from build123d import *

# Parameters (mm, degrees)
BOSS_EXTRUDE1_DEPTH = 2.3
CUT_EXTRUDE1_REACH  = 4.3
SKETCH2_R           = 2.65
SKETCH2_R_2         = 5.125


with BuildPart() as part:
    # Sketch1 → Boss-Extrude1 (new body)
    with BuildSketch(Plane.XY):
        with BuildLine():
            Line((40.15, 0), (-40.15, 0))
            ThreePointArc((-40.15, 0), (-47.221067812, 2.928932188), (-50.15, 10))
            Line((-50.15, 10), (-50.15, 10.4))
            ThreePointArc((-50.15, 10.4), (-47.221067812, 17.471067812), (-40.15, 20.4))
            Line((-40.15, 20.4), (-24.25, 20.4))
            ThreePointArc((-24.25, 20.4), (-20.714466094, 21.864466094), (-19.25, 25.4))
            Line((-19.25, 25.4), (-19.25, 27.1))
            ThreePointArc((-19.25, 27.1), (-20.714466094, 30.635533906), (-24.25, 32.1))
            Line((-24.25, 32.1), (-31.13, 32.1))
            ThreePointArc((-31.13, 32.1), (-34.665533906, 33.564466094), (-36.13, 37.1))
            Line((-36.13, 37.1), (-36.13, 37.6))
            ThreePointArc((-36.13, 37.6), (-34.665533906, 41.135533906), (-31.13, 42.6))
            Line((-31.13, 42.6), (31.13, 42.6))
            ThreePointArc((31.13, 42.6), (34.665533906, 41.135533906), (36.13, 37.6))
            Line((36.13, 37.6), (36.13, 37.1))
            ThreePointArc((36.13, 37.1), (34.665533906, 33.564466094), (31.13, 32.1))
            Line((31.13, 32.1), (24.25, 32.1))
            ThreePointArc((24.25, 32.1), (20.714466094, 30.635533906), (19.25, 27.1))
            Line((19.25, 27.1), (19.25, 25.4))
            ThreePointArc((19.25, 25.4), (20.714466094, 21.864466094), (24.25, 20.4))
            Line((24.25, 20.4), (40.15, 20.4))
            ThreePointArc((40.15, 20.4), (47.221067812, 17.471067812), (50.15, 10.4))
            Line((50.15, 10.4), (50.15, 10))
            ThreePointArc((50.15, 10), (47.221067812, 2.928932188), (40.15, 0))
        make_face()
    extrude(amount=BOSS_EXTRUDE1_DEPTH)

    # Sketch2 → Cut-Extrude1 (cut, up to next)
    with BuildSketch(Plane.XY.offset(2.3), mode=Mode.PRIVATE) as cut_extrude1_sk1:
        with Locations((-40.150797604, 10)):
            Circle(SKETCH2_R)
    cut_extrude1_tool1 = extrude(cut_extrude1_sk1.sketch, amount=-CUT_EXTRUDE1_REACH, mode=Mode.PRIVATE) & part.part
    add(cut_extrude1_tool1.solids().sort_by_distance((-40.150798, 10, 2.3))[0], mode=Mode.SUBTRACT)
    # Sketch2 → Cut-Extrude1 (cut, up to next)
    with BuildSketch(Plane.XY.offset(2.3), mode=Mode.PRIVATE) as cut_extrude1_sk2:
        with Locations((-25.150797604, 10)):
            Circle(SKETCH2_R)
    cut_extrude1_tool2 = extrude(cut_extrude1_sk2.sketch, amount=-CUT_EXTRUDE1_REACH, mode=Mode.PRIVATE) & part.part
    add(cut_extrude1_tool2.solids().sort_by_distance((-25.150798, 10, 2.3))[0], mode=Mode.SUBTRACT)
    # Sketch2 → Cut-Extrude1 (cut, up to next)
    with BuildSketch(Plane.XY.offset(2.3), mode=Mode.PRIVATE) as cut_extrude1_sk3:
        with Locations((0, 21.625)):
            Circle(SKETCH2_R_2)
    cut_extrude1_tool3 = extrude(cut_extrude1_sk3.sketch, amount=-CUT_EXTRUDE1_REACH, mode=Mode.PRIVATE) & part.part
    add(cut_extrude1_tool3.solids().sort_by_distance((0, 21.625, 2.3))[0], mode=Mode.SUBTRACT)
    # Sketch2 → Cut-Extrude1 (cut, up to next)
    with BuildSketch(Plane.XY.offset(2.3), mode=Mode.PRIVATE) as cut_extrude1_sk4:
        with BuildLine():
            Line((23.999202396, 12.65), (26.199202396, 12.65))
            ThreePointArc((26.199202396, 12.65), (28.849202396, 10), (26.199202396, 7.35))
            Line((26.199202396, 7.35), (23.999202396, 7.35))
            ThreePointArc((23.999202396, 7.35), (21.349202396, 10), (23.999202396, 12.65))
        make_face()
    cut_extrude1_tool4 = extrude(cut_extrude1_sk4.sketch, amount=-CUT_EXTRUDE1_REACH, mode=Mode.PRIVATE) & part.part
    add(cut_extrude1_tool4.solids().sort_by_distance((25.099202, 10, 2.3))[0], mode=Mode.SUBTRACT)
    # Sketch2 → Cut-Extrude1 (cut, up to next)
    with BuildSketch(Plane.XY.offset(2.3), mode=Mode.PRIVATE) as cut_extrude1_sk5:
        with BuildLine():
            Line((38.749202396, 12.65), (41.199202396, 12.65))
            ThreePointArc((41.199202396, 12.65), (43.849202396, 10), (41.199202396, 7.35))
            Line((41.199202396, 7.35), (38.749202396, 7.35))
            ThreePointArc((38.749202396, 7.35), (36.099202396, 10), (38.749202396, 12.65))
        make_face()
    cut_extrude1_tool5 = extrude(cut_extrude1_sk5.sketch, amount=-CUT_EXTRUDE1_REACH, mode=Mode.PRIVATE) & part.part
    add(cut_extrude1_tool5.solids().sort_by_distance((39.974202, 10, 2.3))[0], mode=Mode.SUBTRACT)


solid = part.part
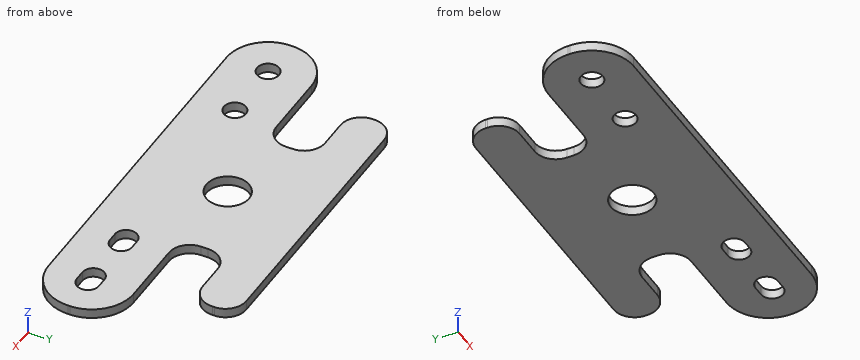
Verification items for the finished model (mm, model axes). Give positions to 0.01 mm unless a question says otherwise; leave off trailing zeros. Order: outer loops, then holes, each group sorted by start corner. A loop starts at its lowest first (then second) coordinate and runs counter-clockwise, first axis right, second up. Notation, with made-up numbers: M 63.5,21.5 L 109.5,21.5 A9 ccw 109.5,25.5 Z; hole C 63.25,63 d7. An arc over 180 degrees is marked long. Answer as a JSON object with one key per item and string values. Group by question number.
1) Cross-section at A-A (x = -39). Enter the section's corners in (y, z), then the cut area to 3 significant figures.
2) Cross-section at C-C (x = 0). Enter the section's corners in (y, z), then the cut area to 3 significant figures.
3) Cross-section at B-B (x = 27.5). Enter the section's corners in (y, z), then the cut area to 3 significant figures.
4) Scan lines: line 1 along Y through (x, z) = (26, 0.3); line 2 along X through (y, z) = (12, 0.85); line 3 along X through (y, z) = (11.5, 2.05). Record each from-to range of solid material in increasing order. Write a range as [from, to].
5) Cross-section at D-D (y = 35). Enter the section's corners in (x, z), then the cut area to 3 significant figures.
6) Depth check by flat-ended pin: pin 1 Ø0.5 at (y, z) = (26.5, 1) entering from +X; pin 2 Ø0.6 at (y, z) = (37.5, 1.5) entering from +X; pin 3 Ø0.9 at (y, z) = (26.5, 1) entering from -X; pin 4 Ø5 at (x, y) = (-40.15, 10) entering from -Z. Enter the tip coordinate at first touch or a pass-through.
Result sheet:
{
 "1": {"outline": "M 0,0 L 7.61,0 L 7.61,2.3 L 0,2.3 Z; M 12.39,0 L 20.4,0 L 20.4,2.3 L 12.39,2.3 Z", "area": "35.9 mm2"},
 "2": {"outline": "M 0,0 L 16.5,0 L 16.5,2.3 L 0,2.3 Z; M 26.75,0 L 42.6,0 L 42.6,2.3 L 26.75,2.3 Z", "area": "74.4 mm2"},
 "3": {"outline": "M 0,0 L 7.69,0 L 7.69,2.3 L 0,2.3 Z; M 12.31,0 L 20.4,0 L 20.4,2.3 L 12.31,2.3 Z; M 32.1,0 L 42.6,0 L 42.6,2.3 L 32.1,2.3 Z", "area": "60.4 mm2"},
 "4": {"line 1": "y = [0, 7.35], [12.65, 20.4], [32.1, 42.6]", "line 2": "x = [-50.02, -41.89], [-38.41, -26.89], [-23.41, 22.26], [27.94, 37.01], [42.94, 50.02]", "line 3": "x = [-50.09, -42.34], [-37.97, -27.34], [-22.97, 21.81], [28.38, 36.56], [43.38, 50.09]"},
 "5": {"outline": "M -35.67,0 L 35.67,0 L 35.67,2.3 L -35.67,2.3 Z", "area": "164 mm2"},
 "6": {"pin 1": "stops at x = 19.25", "pin 2": "stops at x = 36.13", "pin 3": "stops at x = -19.25", "pin 4": "passes through"}
}
